The listing builds one solid part. Answer for the finished solid, in the listing's coordinates (mm). A direction names the side the tool comes from. Give positions to 0.01 mm unless a question says otherwise; leave off trailing zeros. Order: outer loops, then holes, each group sorted by start corner. A loop starts at its lowest first (then second) coordinate and runs counter-clockwise, first axis right, second up.
Autodesk Inventor part; units mm, degrees
ref_plane "YZ Plane" through (0, 0, 0) normal (1, 0, 0) x (0, 1, 0)
ref_plane "XZ Plane" through (0, 0, 0) normal (0, 1, 0) x (-1, 0, 0)
ref_plane "XY Plane" through (0, 0, 0) normal (0, 0, 1) x (1, 0, 0)
sketch "Sketch1" plane through (0, 0, 0) normal (0, 1, 0) x (-1, 0, 0)
  line L0 (0, 0) -> (37, 0)
  line L1 (57, -25.5) -> (57, -44.5)
  line L2 (37, -70) -> (0, -70)
  line L3 (0, -60) -> (0, -10)
  circle A0 centre (27, -20) radius 15 construction
  circle A1 centre (27, -50) radius 15 construction
  circle A2 centre (27, -20) radius 2
  circle A3 centre (27, -50) radius 2
  circle A4 centre (50, -27.5) radius 2
  circle A5 centre (50, -42.5) radius 2
  line L4 (50, -27.5) -> (50, -42.5) construction
  line L5 (27, -20) -> (50, -27.5) construction
  line L6 (25, 0) -> (0, -10)
  line L7 (0, -60) -> (25, -70)
  line L8 (37, 0) -> (57, -15)
  line L9 (57, -55) -> (37, -70)
  line L10 (7, -10) -> (7, -60)
  line L11 (43.6667, -5) -> (12, -5)
  line L12 (43.6667, -65) -> (12, -65)
  line L13 (12, -5) -> (7, -10)
  line L14 (7, -60) -> (12, -65)
  line L15 (32, -5) -> (47.5, -20.5)
  line L16 (47.5, -20.5) -> (52, -20.5)
  line L17 (57, -35) -> (0, -35) construction
  line L18 (32, -65) -> (47.5, -49.5)
  line L19 (47.5, -49.5) -> (52, -49.5)
  line L20 (52, -20.5) -> (57, -25.5)
  line L21 (57, -44.5) -> (52, -49.5)
  point P0 (57, -70)
  point P1 (57, 0)
  point P2 (48, 0)
  point P3 (57, -10)
  point P4 (57, -60)
  point P5 (38, -70)
  point P6 (57, -15)
  point P7 (57, -15)
  point P8 (7, -7.2)
  point P9 (7, -62.8)
  point P10 (7, -5)
  point P11 (7, -65)
  point P12 (7, -5)
  point P13 (7, -65)
  point P14 (57, -20.5)
  point P15 (57, -49.5)
  point P16 (32, -65)
  point P17 (57, -49.5)
  point P18 (57, -20.5)
  point P19 (57, -49.5)
  dimension "d47" = 0
  dimension "d0" = 57
  dimension "d7" = 30
  dimension "d8" = 30
  dimension "d12" = 4
  dimension "d13" = 4
  dimension "d17" = 4
  dimension "d18" = 4
  dimension "d19" = 15
  dimension "d21" = 7
  dimension "d36" = 27.5
  dimension "d38" = 25
  dimension "d40" = 25
  dimension "d52" = 30
  dimension "d90" = 15
  dimension "d91" = 20
  dimension "d92" = 15
  dimension "d93" = 20
  dimension "d124" = 70
  dimension "d132" = 7
  dimension "d133" = 5
  dimension "d134" = 5
  dimension "d135" = 5
  dimension "d136" = 5
  dimension "d137" = 5
  dimension "d138" = 5
  dimension "d139" = 45
  dimension "d140" = 15.5
  dimension "d141" = 7
  dimension "d142" = 5
  dimension "d143" = 5
  dimension "d144" = 5
  dimension "d145" = 5
  dimension "d146" = 25
  dimension "d165" = 15
extrude "Extrusion1" add sketch "Sketch1" along normal blind 3 contours L11 L15 L16 L20 L1 L21 L19 L18 L12 L7 L14 L10 L13 L6 | L6 L13 L11 | L7 L12 L14
sketch "Sketch4" plane through (0, 3, 0) normal (0, 1, 0) x (1, 0, 0)
  line L0 (-33.2, 8.95) -> (-33.2, 41.25)
  line L1 (-33.2, 41.25) -> (-20.8, 41.25)
  line L2 (-20.8, 41.25) -> (-20.8, 8.95)
  line L3 (-20.8, 8.95) -> (-33.2, 8.95)
  line L4 (-33.2, 13.35) -> (-20.8, 13.35)
  line L5 (-33.2, 36.85) -> (-20.8, 36.85)
  circle A0 centre (-27, 20) radius 2.45
  circle A1 centre (-27, 20) radius 2
  circle A2 centre (-27, 20) radius 16.1 construction
  circle A3 centre (-27, 50) radius 2
  circle A4 centre (-27, 50) radius 16.1 construction
  line L6 (-27, 8.95) -> (-27, 13.35) construction
  line L7 (-27, 41.25) -> (-27, 36.85) construction
  circle A5 centre (-27, 10.85) radius 1
  circle A6 centre (-27, 39.35) radius 1
  circle A7 centre (-27, 20) radius 2
  circle A8 centre (-27, 20) radius 9.85 construction
  line L8 (-57, 44.5) -> (-57, 25.5)
  line L9 (-32, 5) -> (-12, 5)
  line L10 (-12, 65) -> (-32, 65)
  line L11 (-12, 5) -> (-10, 7)
  line L12 (-10, 63) -> (-12, 65)
  line L13 (-32, 65) -> (-47.5, 49.5)
  line L14 (-47.5, 49.5) -> (-52, 49.5)
  line L15 (-52, 20.5) -> (-47.5, 20.5)
  line L16 (-47.5, 20.5) -> (-32, 5)
  line L17 (-52, 49.5) -> (-57, 44.5)
  line L18 (-57, 25.5) -> (-52, 20.5)
  line L19 (-10, 7) -> (-10, 63)
  point P0 (0, 0)
  point P1 (-22.9289, 0)
  point P2 (-27.9289, 0)
  dimension "d22" = 32.3
  dimension "d23" = 12.4
  dimension "d24" = 4.4
  dimension "d25" = 4.4
  dimension "d27" = 6.2
  dimension "d28" = 11.05
  dimension "d49" = 32.2
  dimension "d50" = 32.2
  dimension "d53" = 4.9
  dimension "d54" = 2.2
  dimension "d57" = 2
  dimension "d58" = 2
  dimension "d59" = 1.9
  dimension "d60" = 1.9
  dimension "d87" = 19.7
sketch "Sketch10" plane through (0, 3, 0) normal (0, 1, 0) x (1, 0, 0)
  line L0 (-12, 5) -> (-7, 10)
  line L1 (-10, 7) -> (-10, 63)
  line L2 (-7, 60) -> (-12, 65)
  line L3 (-7, 10) -> (-7, 60)
  line L4 (-7, 60) -> (-12, 65)
  line L5 (-47.5, 20.5) -> (-32, 5)
  line L6 (-32, 65) -> (-47.5, 49.5)
  line L7 (-32, 5) -> (-12, 5)
  line L8 (-12, 65) -> (-32, 65)
  line L9 (-12, 65) -> (-32, 65)
  point P0 (0, 0)
  dimension "d147" = 3
extrude "Extrusion7" add sketch "Sketch10" along normal blind 15.1
sketch "Sketch11" plane through (0, 18.1, 0) normal (0, 1, 0) x (1, 0, 0)
  line L0 (-12, 5) -> (-10, 7)
  line L1 (-10, 7) -> (-30, 7)
  line L2 (-35, 12) -> (-35, 58.0775)
  line L3 (-30, 63.0775) -> (-10, 63.0775)
  line L4 (-10, 63.0775) -> (-10, 7)
  line L5 (-30, 7) -> (-35, 12)
  line L6 (-35, 58.0775) -> (-30, 63.0775)
  circle A0 centre (-27, 10.85) radius 1
  circle A1 centre (-27, 39.35) radius 1
  line L7 (-20.8, 8.95) -> (-33.2, 8.95)
  line L8 (-33.2, 8.95) -> (-33.2, 41.25)
  line L9 (-33.2, 36.85) -> (-20.8, 36.85)
  line L10 (-33.2, 41.25) -> (-20.8, 41.25)
  line L11 (-20.8, 41.25) -> (-20.8, 8.95)
  line L12 (-33.2, 13.35) -> (-20.8, 13.35)
  circle A2 centre (-27, 50) radius 2
  circle A3 centre (-27, 50) radius 4
  point P0 (0, 0)
  point P1 (-35, 63.0775)
  point P2 (-35, 7)
  dimension "d150" = 25
  dimension "d151" = 56.0775
  dimension "d152" = 5
  dimension "d153" = 5
  dimension "d154" = 5
  dimension "d155" = 5
  dimension "d156" = 8
extrude "Extrusion8" add sketch "Sketch11" against normal blind 3 contours L1 L5 L7 L11 L10 L8 L2 L6 L3 L4 | L5 L8 L12 L11 L7 | L8 L10 L11 L9
properties part number "base 2.0 upload"
1) Straight lines are drawn through the part: probe 1 along Z at (x, y) = (-50, 2.35); probe 2 along Z at (x, y) = (-27, 15.95); probe 3 along Z at (x, y) = (-27, 1.25). For each, find the intervals that lie inside material, in ascending order.
Geometry says:
probe 1: z = -49.5 to -44.5, -40.5 to -29.5, -25.5 to -20.5
probe 2: z = -63.08 to -54, -46 to -40.35, -38.35 to -36.85, -13.35 to -11.85, -9.85 to -7
probe 3: z = -65 to -52, -48 to -22, -18 to -5
2) A tool of negligible diameter and unlimited length cuts with its end or side. For faces 4 (the flat face through (-20, 17, -63.078)), 5 (the flat face through (-32.535, 16.621, -60.543)), 6 (the flat face through (-10, 9, -35)), 7 (the cylindrical face through (-27.13, 16.62, -40.34)), 8 (the flat face through (-20, 17, -7)), from which of +Z, -Z, +X, -X, +Y, -Y can it reach the whole face along a straight path? Write none if from no direction.
Geometry says:
face 4: -Z, +X, -X, +Y
face 5: -Z, -X, +Y
face 6: +Z, -Z, -X
face 7: +Y
face 8: +Z, +X, -X, +Y
3) Find section A-A (z = -39.35). Write down the section's boundary in (x, y), then the cut area to 3 significant figures.
Geometry says:
outline: (-57, 0) - (-7, 0) - (-7, 18.1) - (-26, 18.1) - (-26, 15.1) - (-10, 15.1) - (-10, 3) - (-57, 3) - close; (-35, 15.1) - (-28, 15.1) - (-28, 18.1) - (-35, 18.1) - close
area: 264 mm2
4) Find section B-B (z = -27.5). Write down the section's boundary in (x, y).
Geometry says:
outline: (-57, 0) - (-52, 0) - (-52, 3) - (-57, 3) - close; (-48, 0) - (-7, 0) - (-7, 18.1) - (-20.8, 18.1) - (-20.8, 15.1) - (-10, 15.1) - (-10, 3) - (-48, 3) - close; (-35, 15.1) - (-33.2, 15.1) - (-33.2, 18.1) - (-35, 18.1) - close
5) Find section D-D (x = -18). Write down the section's boundary in (y, z), then the cut area to 3 significant figures.
Geometry says:
outline: (0, -65) - (3, -65) - (3, -5) - (0, -5) - close; (15.1, -63.08) - (18.1, -63.08) - (18.1, -7) - (15.1, -7) - close
area: 348 mm2
6) Given P1, Ø7, axis at x = -27, z = -50, coming from the -Y side; P2, Ø2.5, axis at x = -50, y = 2, coming from the +Z side; P3, Ø1, axis at x = -42.5, y = 2, coming from the +Z side; P4, Ø0.9, axis at x = -48.5, y = 2, coming from the -Z side, each flat-ended and moving along its own axis, determine where each tip first touches the part or whether it passes through.
Geometry says:
P1: stops at y = 0
P2: stops at z = -20.5
P3: stops at z = -15
P4: stops at z = -49.5
7) For a pull along Z with two mould halves and no side action, classify faces 1 (the flat face through (-40, 1, -13)), 2 (the flat face through (-57, 1, -35)), 3 (the flat face through (-27, 17, -36.85)) as +Z half, -Z half, draft (parallel to the pull), parting line (faces both ways), or undercut.
Geometry says:
face 1: +Z half
face 2: draft
face 3: undercut
8) Find section C-C (x = -50). Write down the section's boundary in (y, z).
Geometry says:
outline: (0, -49.5) - (3, -49.5) - (3, -44.5) - (0, -44.5) - close; (0, -40.5) - (3, -40.5) - (3, -29.5) - (0, -29.5) - close; (0, -25.5) - (3, -25.5) - (3, -20.5) - (0, -20.5) - close
